```python
from build123d import *

# Parameters (mm, degrees)
CROQUIS1_R              = 10
SALIENTE_EXTRUIR1_DEPTH = 18


with BuildPart() as part:
    # Croquis1 → Saliente-Extruir1 (new body)
    with BuildSketch(Plane.XY):
        with BuildLine():
            Line((0, 0), (0, 70))
            Line((0, 70), (11, 70))
            Line((11, 70), (11, 64.196152423))
            ThreePointArc((11, 64.196152423), (8.204445042, 57.447085729), (14, 53))
            Line((14, 53), (48.5, 53))
            ThreePointArc((48.5, 53), (54.295554958, 57.447085729), (51.5, 64.196152423))
            Line((51.5, 64.196152423), (51.5, 70))
            Line((51.5, 70), (83.5, 70))
            Line((83.5, 70), (83.5, 64.196152423))
            ThreePointArc((83.5, 64.196152423), (80.704445042, 57.447085729), (86.5, 53))
            Line((86.5, 53), (121, 53))
            ThreePointArc((121, 53), (126.795554958, 57.447085729), (124, 64.196152423))
            Line((124, 64.196152423), (124, 70))
            Line((124, 70), (135, 70))
            Line((135, 70), (135, 0))
            Line((135, 0), (0, 0))
        make_face()
        with Locations((67.5, 53)):
            Circle(CROQUIS1_R, mode=Mode.SUBTRACT)
    extrude(amount=SALIENTE_EXTRUIR1_DEPTH)


solid = part.part
```
Work out the finished part from the listing and answer in its coordinate system (mm). A direction names the side the tool comes from. Give positions to 0.01 mm unless a question says otherwise; leave off trailing zeros. Loops run counter-clockwise (first coordinate to the right, second up) from the corner with the lowest first, then second, coordinate; pieces in that order, holes last. Notation, with made-up numbers: (-13.5, 13) -> (-5.5, 13) arc R18 cw to (-5.5, 43) -> close; hole circle Ø3 at (-7.5, 74). An arc over 180 degrees is marked (long way). Write item = value, one per line. Start each with the question number.
(1) Find section B-B on z = 8.25. Give the vertices of the cut face in (x, y).
(2) Find section A-A on x = 75.5. Give the vertices of the cut face in (y, z), and give its area (3 significant figures).
(3) Find section C-C on y = 57. Give the vertices of the cut face in (x, z).
(4) Find section D-D on x = 36. Give the vertices of the cut face in (y, z).
(5) Find the intervals of material crossed by probe 1 along X at (y, z) = (67.5, 8.5); probe 2 along Y at (x, z) = (67.5, 13.75); probe 3 along Y at (x, z) = (95, 1.25), in increasing order. Write a range as from..to.
(6) Given pin 1 Ø6 at (x, z) = (117, 4.5) entering from +Y; pin 2 Ø12 at (x, y) = (67.5, 53) entering from -Z, each flat-ended and moving along its own axis, determine where each tip first touches the part or whether it passes through.
(7) Which of the six approach directions +Z, -Z, +X, -X, +Y, -Y give full straight-line access (tool end or side, diameter ignored) to faces 1 (the cylindrical face through (8.177, 57.554, 8.874)), 2 (the flat face through (0, 35, 9)), 3 (the flat face through (104, 53, 9))?
(8) The mould has two halves that part along X. Classify faces 4 (the flat face through (135, 35, 9)), 5 (the cylindrical face through (59.56, 46.92, 8.87)), 6 (the flat face through (31, 53, 9)), 7 (the flat face through (68, 0, 9)): +X half, -X half, draft (parallel to the pull), parting line (faces both ways), or undercut.
From the geometry:
q1.outline = (0, 0) -> (135, 0) -> (135, 70) -> (124, 70) -> (124, 64.2) arc R6 cw to (121, 53) -> (86.5, 53) arc R6 cw to (83.5, 64.2) -> (83.5, 70) -> (51.5, 70) -> (51.5, 64.2) arc R6 cw to (48.5, 53) -> (14, 53) arc R6 cw to (11, 64.2) -> (11, 70) -> (0, 70) -> close; hole circle Ø20 at (67.5, 53)
q2.outline = (0, 0) -> (47, 0) -> (47, 18) -> (0, 18) -> close; (59, 0) -> (70, 0) -> (70, 18) -> (59, 18) -> close
q2.area = 1,040 mm^2
q3.outline = (0, 0) -> (8.34, 0) -> (8.34, 18) -> (0, 18) -> close; (54.16, 0) -> (58.33, 0) -> (58.33, 18) -> (54.16, 18) -> close; (76.67, 0) -> (80.84, 0) -> (80.84, 18) -> (76.67, 18) -> close; (126.66, 0) -> (135, 0) -> (135, 18) -> (126.66, 18) -> close
q4.outline = (0, 0) -> (53, 0) -> (53, 18) -> (0, 18) -> close
q5.probe_1 = 0..11, 51.5..83.5, 124..135
q5.probe_2 = 0..43, 63..70
q5.probe_3 = 0..53
q6.pin_1 = 53
q6.pin_2 = through
q7.face_1 = +Z, -Z
q7.face_2 = +Z, -Z, -X, +Y, -Y
q7.face_3 = +Z, -Z, +Y
q8.face_4 = +X half
q8.face_5 = undercut
q8.face_6 = undercut
q8.face_7 = draft
